from build123d import *

# Parameters (mm, degrees)
F1_DEPTH = 13.716
F2_R     = 6.8579
F3_R     = 2.54
F4_DEPTH = 5.5678543904


# Not quite as in the source:
# - a fillet or chamfer is up to 0.001 mm smaller than in the source, because OpenCascade refuses the exact size


with BuildPart() as f1:
    # F0 (on Front) → F1 (new body)
    with BuildSketch(Plane.XZ):
        with BuildLine():
            ThreePointArc((-10.6891457096, -6.858), (-12.7, 0), (-10.6891457096, 6.858))
            Line((-10.6891457096, 6.858), (-16.256, 6.858))
            Line((-16.256, 6.858), (-16.256, 0))
            Line((-16.256, 0), (-16.256, -6.858))
            Line((-16.256, -6.858), (-10.6891457096, -6.858))
        make_face()
    extrude(amount=F1_DEPTH)

    # F2 (radius 6.858 in the source; OpenCascade refuses exactly that, so slightly less here)
    f2_edges = [f1.edges().sort_by_distance(p)[0] for p in [
        (-13.472573, 0, 6.858),
        (-13.472573, -13.716, 6.858),
        (-13.472573, -13.716, -6.858),
        (-13.472573, 0, -6.858),
    ]]
    fillet(f2_edges, radius=F2_R)

    # F3 (on face) → F4 (cut, through all)
    with BuildSketch(Plane(origin=(-16.256, 0, 0), x_dir=(0, -1, 0), z_dir=(-1, 0, 0))):
        with Locations((6.858, 0)):
            Circle(F3_R)
    extrude(amount=-F4_DEPTH, mode=Mode.SUBTRACT)


solid = f1.part
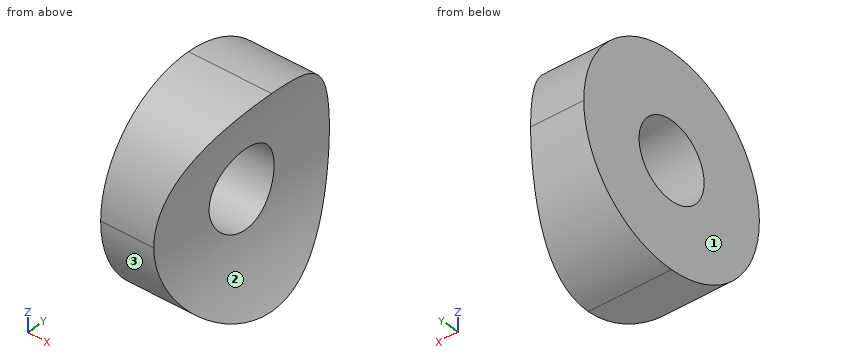
Work out the finished part from the listing and answer in its coordinate system (mm). Face numbers are marked on the shaded views. Round coordinates to 2 decimals unless told otherwise and drop trailing zeros. Loops run counter-clockwise (first coordinate to the right, second up) from the corner with the lowest first, then second, coordinate; pieces in that order, holes last. Notation, with made-up numbers: M 49,89.25 L 102,89.25 A28 ccw 102,125.25 Z; hole C 37,-30.5 d6. An arc over 180 degrees is marked long. One line per question, with ' | ' between items. Start each with the question number.
(1) A cutting plane is placed at B-B on y = -4.5. Write down the section's boundary in (x, z), plus the area to 3 significant figures.
(2) Find the intervals of material crossed by line 1 (Y direction, x = -13.75, z = 0); line 2 (Z direction, x = -13.7, y = -6); line 3 (Z direction, x = -14.2, y = -9), in increasing order.
(3) Flat-ended cylindrical pins translate along their axes: pin 1 Ø3 at (x, y) = (-15, -7.5) entering from -Z; pin 2 Ø2 at (y, z) = (-10.5, 1.5) entering from +X; pin 3 Ø1 at (x, y) = (-15, -3.5) entering from +Z; pin 4 Ø1 at (x, y) = (-12, -2.5) entering from -Z. Find the tip coordinate at first contact, or state that the pin passes through.
(4) For a pull along Z with two mould halves and no side action, classify the marked faces 1, 2 and 3 as released by +Z, released by -Z, zero draft, split by the parting line, or undercut.
(5) A cutting plane is placed at D-D on z = -3. Write down the section's boundary in (x, y), plus the area to 3 significant figures.
Geometry check:
1) outline: M -16.26,-6.44 L -10.95,-6.44 A12.7 cw -12.66,-0.94 L -16.26,-0.94 Z; M -16.26,0.94 L -12.66,0.94 A12.7 cw -10.95,6.44 L -16.26,6.44 Z | area: 46.4 mm²
2) line 1: y = -13.72 to -9.4, -4.32 to 0 | line 2: z = -6.8 to -2.39, 2.39 to 6.8 | line 3: z = -6.51 to -1.37, 1.37 to 6.51
3) pin 1: stops at z = -6.86 | pin 2: stops at x = -12.45 | pin 3: stops at z = 6.23 | pin 4: stops at z = -5.67
4) face 1: zero draft | face 2: undercut | face 3: released by -Z
5) outline: M -16.26,-13.03 L -12.34,-13.03 L -12.34,-0.69 L -16.26,-0.69 Z | area: 48.3 mm²
